Geometry: see drawing. Coordinates: mm, zero at the bounding-box minimum. Coordinates: 2 decimals unless noted, no trailing zeros. Order: outer loops, then holes, each group sorted by start corner. A loop starts at its lowest first (then second) coordinate and runs counter-clockwise, first axis right, second up. Notation, with made-up numbers: (9, -24.5) -> (40, -24.5) arc R37 ccw to (40, 13.5) -> close; hole circle Ø8 at (11, 78). An arc over 180 degrees is marked (long way). Use one line per item in the form item = value.
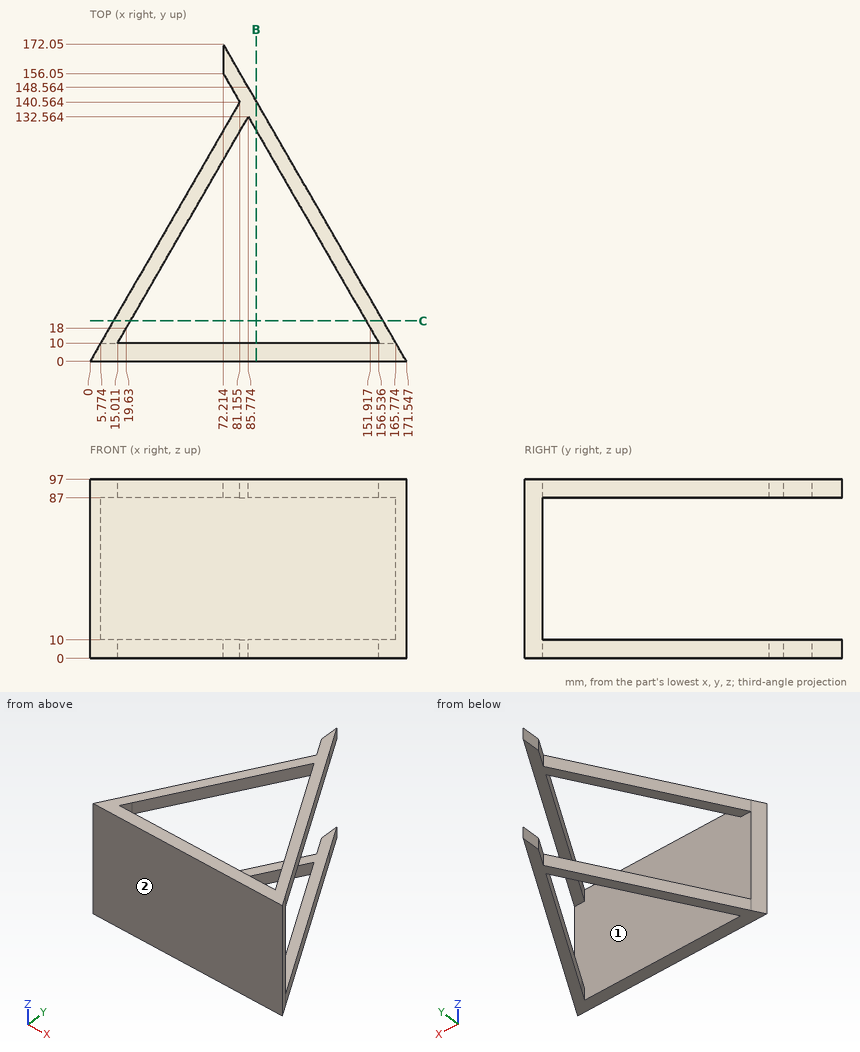
1) Contact query for flat-ended pins moving along their axis: P1, Ø4, axis at y = 120.5, z = 86.5, coming from the -X side; P2, Ø3, axis at y = 167, z = 6, coming from the -X side; P3, Ø4, axis at y = 109.5, z = 86.5, coming from the +X side (1 decimal); P4, Ø5, axis at x = 32, y = 34, coming from the +Z side. Output: stop coordinate, or through.
Results found:
P1 = 68.45
P2 = 72.21
P3 = 109.4
P4 = through
2) Material intervals for probe 1 along Z at (x, y) = (76, 121); probe 2 along Y at (x, z) = (39.5, 26.5); probe 3 along Y at (x, z) = (20, 9) (1 decimal), sorted ascending. Write a range as from..to.
Results found:
probe_1 = 0..10, 87..97
probe_2 = 0..10
probe_3 = 0..10, 18.6..34.6
3) Section C-C, the plane y = 22. Output: boundary loops of the cut face in (x, z) (1 decimal).
Results found:
outline = (12.7, 0) -> (21.9, 0) -> (21.9, 10) -> (12.7, 10) -> close; (12.7, 87) -> (21.9, 87) -> (21.9, 97) -> (12.7, 97) -> close; (149.6, 0) -> (158.8, 0) -> (158.8, 10) -> (149.6, 10) -> close; (149.6, 87) -> (158.8, 87) -> (158.8, 97) -> (149.6, 97) -> close
4) Section B-B, the plane x = 90. Output: boundary loops of the cut face in (y, z).
Results found:
outline = (0, 0) -> (10, 0) -> (10, 97) -> (0, 97) -> close; (125.24, 0) -> (141.24, 0) -> (141.24, 10) -> (125.24, 10) -> close; (125.24, 87) -> (141.24, 87) -> (141.24, 97) -> (125.24, 97) -> close
5) Pull-direction query (X, two-part tool) for the marked faces 1 and 2; classes: released by +X, released by -X, zero draft, split by the parting line, or undercut.
Results found:
face_1 = undercut
face_2 = zero draft
